from build123d import *

# Parameters (mm, degrees)
EXTRUDE_1_DEPTH      = 10
SKETCH_3_R           = 2
CUT_EXTRUDE_3_DEPTH  = 10
CUT_EXTRUDE_19_DEPTH = 10
SKETCH_15_R          = 2
CUT_EXTRUDE_20_DEPTH = 10


with BuildPart() as part:
    # Эскиз1 → Бобышка-Вытянуть1 (new body)
    with BuildSketch(Plane(origin=(0, 0, 0), x_dir=(1, 0, 0), z_dir=(0, 1, 0))):
        with BuildLine():
            Line((0, 1), (0, 14))
            ThreePointArc((0, 14), (0.292893219, 14.707106781), (1, 15))
            Line((1, 15), (9, 15))
            ThreePointArc((9, 15), (9.707106781, 14.707106781), (10, 14))
            Line((10, 14), (10, 1))
            add(Edge.make_bspline(
                [(9, 1), (9.166666667, 0.5), (9.5, -0.5), (9.833333333, 0.5), (10, 1)],
                knots=[0, 0, 0, 0, 0.5, 1, 1, 1, 1], degree=3))
            Line((9, 1), (9, 13))
            ThreePointArc((9, 13), (8.707106781, 13.707106781), (8, 14))
            Line((8, 14), (2, 14))
            ThreePointArc((2, 14), (1.292893219, 13.707106781), (1, 13))
            Line((1, 13), (1, 1))
            add(Edge.make_bspline(
                [(0, 1), (0.5, -1), (1, 1)],
                knots=[0, 0, 0, 1, 1, 1], degree=2))
        make_face()
    extrude(amount=EXTRUDE_1_DEPTH)

    # Эскиз3 → Вырез-Вытянуть3 (cut)
    with BuildSketch(Plane(origin=(10, 0, 0), x_dir=(0, 0, -1), z_dir=(1, 0, 0))):
        with Locations((5, 5)):
            Circle(SKETCH_3_R)
    extrude(amount=-CUT_EXTRUDE_3_DEPTH, mode=Mode.SUBTRACT)

    # Эскиз14 → Вырез-Вытянуть19 (cut)
    with BuildSketch(Plane(origin=(0, 0, 0), x_dir=(0, 0, -1), z_dir=(1, 0, 0))):
        with BuildLine():
            Line((5, 10), (0, 10))
            Line((0, 10), (0, 0))
            Line((0, 0), (5, 0))
            ThreePointArc((5, 0), (0.246325104, 5), (5, 10))
        make_face()
    extrude(amount=CUT_EXTRUDE_19_DEPTH, mode=Mode.SUBTRACT)

    # Эскиз15 → Вырез-Вытянуть20 (cut)
    with BuildSketch(Plane(origin=(0, 0, -15), x_dir=(-1, 0, 0), z_dir=(0, 0, -1))):
        with Locations((-5, 5)):
            Circle(SKETCH_15_R)
    extrude(amount=-CUT_EXTRUDE_20_DEPTH, mode=Mode.SUBTRACT)


solid = part.part
The listing builds one solid part. Answer for the finished solid, in the listing's coordinates (mm). A direction names the side the tool comes from. Coordinates: 2 decimals unless noted, no trailing zeros. Write each loop counter-clockwise with the first axis right and the second up, starting at its lowest first coordinate (ties: lowest second). Pieces come first, ordered by that corner, then holes. Notation, with made-up numbers: (3, 2.5) - (10, 2.5) arc R16 cw to (10, 10.5) - close; hole circle Ø7 at (-1.75, 4.25). An arc over 180 degrees is marked (long way). Put each result on its own line as item: value.
1. The part is cut by section B-B on x = 5. Give the vertices of the cut face in (y, z).
Answer sheet:
outline: (0, -15) - (3, -15) - (3, -14) - (0, -14) - close; (7, -15) - (10, -15) - (10, -14) - (7, -14) - close
2. Flat-ended cylindrical pins translate along their axes: pin 1 Ø5 at (x, y) = (5, 5) entering from -Z; pin 2 Ø2 at (x, z) = (3, -9) entering from -Y; pin 3 Ø1.8 at (x, y) = (4, 2.5) entering from +Z. Find the tip coordinate at first contact, or state that the pin passes through.
Answer sheet:
pin 1: stops at z = -15
pin 2: passes through
pin 3: stops at z = -14
3. Find the intervals of material crossed by line 1 along Y through (x, z) = (0.2, -5); line 2 along X through (y, z) = (8.5, -13); line 3 along Z through (x, y) = (7, 8.25), in increasing order. Write a range as from..to.
Answer sheet:
line 1: y = 0..3, 7..10
line 2: x = 0..1, 9..10
line 3: z = -15..-14
4. The part is cut by section D-D on x = 0.5. Give the vertices of the cut face in (y, z), plus the area to 3 significant figures.
Answer sheet:
outline: (0, -14.87) - (10, -14.87) - (10, -5) arc R5.01 ccw to (0, -5) - close; hole circle Ø4 at (5, -5)
area: 123 mm^2
5. Determine the mould class of faces 1 (the face through (0.493, 4.893, -0.247)), 2 (the face through (10, 5, -8)), 3 (the face through (6.998, 5.088, -14.507)) for opening direction Y: pulls with the +Y half, pulls with the -Y half, needs draft (parallel to the pull), parting line crosses it, or undercut.
Answer sheet:
face 1: parting line crosses it
face 2: needs draft
face 3: undercut
6. A tool of negligible diameter and unlimited length cuts with its end or side. For faces 4 (the face through (0, 4.9, -7.4)), 5 (the face through (5, 2.7, -14)), from which of +Z, -Z, +X, -X, +Y, -Y can it reach the whole face along a straight path? Write none if from no direction.
Answer sheet:
face 4: +Z, -Z, -X, +Y, -Y
face 5: +Z, +Y, -Y
7. The part is cut by section C-C on y = 5. State how many separate pieces and enclosed holes the cut face has, plus the area to 3 significant figures.
Answer sheet:
separate pieces: 4
enclosed holes: 0
area: 25.1 mm^2
8. The part is cut by section A-A on z = -10.25. Give the vertices of the cut face in (x, y).
Answer sheet:
outline: (0, 0) - (1, 0) - (1, 10) - (0, 10) - close; (9, 0) - (10, 0) - (10, 10) - (9, 10) - close
